The listing builds one solid part. Answer for the finished solid, in the listing's coordinates (mm). A direction names the side the tool comes from. Coordinates: 2 decimals unless noted, no trailing zeros. Order: outer loops, then holes, each group sorted by start corner. A loop starts at its lowest first (then second) coordinate and runs counter-clockwise, first axis right, second up. Notation, with made-up numbers: (-27.75, 28.25) -> (-18.75, 28.25) arc R10 cw to (-18.75, 40.25) -> close; hole circle Ø6 at (-2, 17.25). An arc over 180 degrees is marked (long way). Answer in a Markdown table with one row per item.
```python
from build123d import *

# Parameters (mm, degrees)
TAP_DRILL_FOR_1_4_20_TAP2_AT_2_COUNT = 2
TAP_DRILL_FOR_1_4_20_TAP2_AT_2_PITCH = 43.780544641
TAP_DRILL_FOR_1_4_20_TAP2_AT_3_COUNT = 2
TAP_DRILL_FOR_1_4_20_TAP2_AT_3_PITCH = 61.91504
TAP_DRILL_FOR_1_4_20_TAP2_AT_4_COUNT = 2
TAP_DRILL_FOR_1_4_20_TAP2_AT_4_PITCH = 43.780544641


with BuildPart() as part:
    # Housing Sketch → Housing Revolve (revolve)
    with BuildSketch(Plane(origin=(0, 0, 0), x_dir=(0, 0, -1), z_dir=(1, 0, 0)), mode=Mode.PRIVATE) as housing_revolve_sk:
        Polygon((83.82, 36.5125), (0, 36.5125), (0, 21), (22, 21), (22, 18), (55.945, 18), (55.945, 21), (83.82, 21), align=None)
    revolve(housing_revolve_sk.sketch.rotate(Axis((0, 0, -141.5522592), (0, 0, 1)), 90), axis=Axis((0, 0, -141.5522592), (0, 0, 1)))

    # Sketch8 → Tap Drill for 1/4-20 Tap2 (revolve, cut)
    with BuildSketch(Plane(origin=(0, 30.95752, 0), x_dir=(0, -1, 0), z_dir=(1, 0, 0))):
        Polygon((0, 0), (0, 14.233816902), (2.5527, 12.7), (2.5527, 0), align=None)
    tap_drill_for_1_4_20_tap2 = revolve(axis=Axis((0, 30.95752, 6.35), (0, 0, -1)), mode=Mode.SUBTRACT)

    # Tap Drill for 1/4-20 Tap2 at 2: Tap Drill for 1/4-20 Tap2 ×2
    with Locations(*[Vector(0.7071067811865476, -0.7071067811865476, 0) * (i * TAP_DRILL_FOR_1_4_20_TAP2_AT_2_PITCH) for i in range(1, TAP_DRILL_FOR_1_4_20_TAP2_AT_2_COUNT)]):
        add(tap_drill_for_1_4_20_tap2, mode=Mode.SUBTRACT)

    # Tap Drill for 1/4-20 Tap2 at 3: Tap Drill for 1/4-20 Tap2 ×2
    with Locations(*[(0, -i * TAP_DRILL_FOR_1_4_20_TAP2_AT_3_PITCH, 0) for i in range(1, TAP_DRILL_FOR_1_4_20_TAP2_AT_3_COUNT)]):
        add(tap_drill_for_1_4_20_tap2, mode=Mode.SUBTRACT)

    # Tap Drill for 1/4-20 Tap2 at 4: Tap Drill for 1/4-20 Tap2 ×2
    with Locations(*[Vector(-0.7071067811865476, -0.7071067811865476, 0) * (i * TAP_DRILL_FOR_1_4_20_TAP2_AT_4_PITCH) for i in range(1, TAP_DRILL_FOR_1_4_20_TAP2_AT_4_COUNT)]):
        add(tap_drill_for_1_4_20_tap2, mode=Mode.SUBTRACT)

    # Mirror1: Tap Drill for 1/4-20 Tap2 across plane
    add(tap_drill_for_1_4_20_tap2.mirror(Plane(origin=(0, 0, -41.91), x_dir=(1, 0, 0), z_dir=(0, 0, -1))), mode=Mode.SUBTRACT)

    # Mirror1 copy 1 sketch → Mirror1 copy 1 (revolve, cut)
    with BuildSketch(Plane(origin=(30.95752, 0, -83.82), x_dir=(0, -1, 0), z_dir=(1, 0, 0))):
        Polygon((0, 0), (0, -14.233816902), (2.5527, -12.7), (2.5527, 0), align=None)
    revolve(axis=Axis((30.95752, 0, -90.17), (0, 0, -1)), mode=Mode.SUBTRACT)

    # Mirror1 copy 2 sketch → Mirror1 copy 2 (revolve, cut)
    with BuildSketch(Plane(origin=(0, -30.95752, -83.82), x_dir=(0, -1, 0), z_dir=(1, 0, 0))):
        Polygon((0, 0), (0, -14.233816902), (2.5527, -12.7), (2.5527, 0), align=None)
    revolve(axis=Axis((0, -30.95752, -90.17), (0, 0, -1)), mode=Mode.SUBTRACT)

    # Mirror1 copy 3 sketch → Mirror1 copy 3 (revolve, cut)
    with BuildSketch(Plane(origin=(-30.95752, 0, -83.82), x_dir=(0, -1, 0), z_dir=(1, 0, 0))):
        Polygon((0, 0), (0, -14.233816902), (2.5527, -12.7), (2.5527, 0), align=None)
    revolve(axis=Axis((-30.95752, 0, -90.17), (0, 0, -1)), mode=Mode.SUBTRACT)


solid = part.part
```
(1) Which of the six approach directions +Z, -Z, +X, -X, +Y, -Y give full straight-line access (tool end or side, diameter ignored) to faces 1 (the cylindrical face through (13.267, -12.165, -39.21)), 2 (the cylindrical face through (-20.03, -6.31, -11.15)), 3 (the cylindrical face through (28.427, 0.332, -77.559))?
Check values:
| item | result |
|---|---|
| face 1 | +Z, -Z |
| face 2 | +Z |
| face 3 | -Z |
(2) For a pull along X with two mould halves and no side action, classify faces 4 (the cylindrical face through (28.427, 0.332, -6.261)), 5 (the conical face through (-0.02, 31.4, -13.97)), 6 (the flat face through (16, 16, -83.82)) as released by +X, released by -X, zero draft, split by the parting line, or undercut.
Check values:
| item | result |
|---|---|
| face 4 | undercut |
| face 5 | undercut |
| face 6 | zero draft |
(3) Find the intervals of material crossed by line 1 along Y through (x, z) = (0, -65); line 2 along Y through (x, z) = (0, -43); line 3 along X through (y, z) = (8.5, -23.5), in increasing order. Write a range as from..to.
Check values:
| item | result |
|---|---|
| line 1 | -36.51..-21, 21..36.51 |
| line 2 | -36.51..-18, 18..36.51 |
| line 3 | -35.51..-15.87, 15.87..35.51 |
(4) A cutting plane is placed at A-A, the plane x = -12. Determine the outline of the cut face in (y, z) (3 decimals).
Check values:
| item | result |
|---|---|
| outline | (-34.484, -83.82) -> (-17.234, -83.82) -> (-17.234, -55.945) -> (-13.416, -55.945) -> (-13.416, -22) -> (-17.234, -22) -> (-17.234, 0) -> (-34.484, 0) -> close; (13.416, -55.945) -> (17.234, -55.945) -> (17.234, -83.82) -> (34.484, -83.82) -> (34.484, 0) -> (17.234, 0) -> (17.234, -22) -> (13.416, -22) -> close |
(5) Flat-ended cylindrical pins translate along their axes: pin 1 (2 mm diameter, centred on y = 22, z = -45.5, fed in from -X); pin 2 (12 mm diameter, centred on x = 16, z = -17.5, fed in from -Y); pin 3 (25 mm diameter, centred on x = 0, y = 0, fed in from -Z); pin 4 (10 mm diameter, centred on x = -25, z = -43.5, fed in from +Y). Find the tip coordinate at first contact, or state that the pin passes through.
Check values:
| item | result |
|---|---|
| pin 1 | x = -29.87 |
| pin 2 | y = -35.12 |
| pin 3 | through |
| pin 4 | y = 30.55 |
(6) A cutting plane is placed at C-C, the plane z = -50. Determine the outline of the cut face in (x, y) (1 decimal), then the cut area to 3 significant figures.
Check values:
| item | result |
|---|---|
| outline | circle Ø73 at (0, 0); hole circle Ø36 at (0, 0) |
| area | 3,170 mm² |
(7) A cutting plane is placed at D-D, the plane z = -11. Determine the outline of the cut face in (x, y) (1 decimal).
Check values:
| item | result |
|---|---|
| outline | circle Ø73 at (0, 0); hole circle Ø5.1 at (-31, 0); hole circle Ø42 at (0, 0); hole circle Ø5.1 at (0, -31); hole circle Ø5.1 at (0, 31); hole circle Ø5.1 at (31, 0) |
(8) A cutting plane is placed at B-B, the plane y = 15. Determine the outline of the cut face in (x, z) (3 decimals).
Check values:
| item | result |
|---|---|
| outline | (-33.289, -83.82) -> (-14.697, -83.82) -> (-14.697, -55.945) -> (-9.95, -55.945) -> (-9.95, -22) -> (-14.697, -22) -> (-14.697, 0) -> (-33.289, 0) -> close; (9.95, -55.945) -> (14.697, -55.945) -> (14.697, -83.82) -> (33.289, -83.82) -> (33.289, 0) -> (14.697, 0) -> (14.697, -22) -> (9.95, -22) -> close |
